Build history of the part. All positions in model axes, mm. Give positions to 0.01 mm unless a question says otherwise; leave off trailing zeros. Order: outer loops, then holes, each group sorted by start corner. A loop starts at its lowest first (then second) coordinate and runs counter-clockwise, first axis right, second up. Notation, with made-up numbers: (-22.5, -2.75) - (-1.5, -2.75) arc R27 ccw to (-1.5, 26.25) - close; hole circle Ø8 at (21.25, 11). An arc over 180 degrees is marked (long way). Use a Markdown table: item, result. Add a question column.
(1) Wall check: line 1 (X direction, y = 2.3, z = -2.5); line 2 (X direction, y = 2.25, z = -3); line 3 (Z direction, x = 6.75, y = 1.65). Give the ranges that are in metal, low to high.
(2) Slice it at D-D (x = 3). Write the cut outline in (y, z).
(3) Slice it at B-B (y = 2.6). Write the cut outline in (x, z) (3 decimals), then the cut area to 3 significant figures.
(4) Slice it at C-C (z = -13). Write the cut outline in (x, y).
(5) Mould opens along X. For faces 1 (the face through (1.44, 1.48, -2.85)), 2 (the face through (2.095, 1.479, -10.248)), 3 (the face through (7, 1, 0)) say: +X half, -X half, draft (parallel to the pull), parting line (faces both ways), or undercut.
(6) Slice it at A-A (z = -2.5). Write the cut outline in (x, y).
from build123d import *

# Parameters (mm, degrees)
SKETCH1_R           = 1.6
SKETCH1_R_2         = 4
BOSS_EXTRUDE1_DEPTH = 3
FILLET1_R           = 5


with BuildPart() as part:
    # Sketch1 → Boss-Extrude1 (new body)
    # profile 1 of 2: a face of its own
    with BuildSketch(Plane(origin=(0, 0, 0), x_dir=(1, 0, 0), z_dir=(0, 1, 0))):
        with BuildLine():
            Line((0, 5), (0, 0))
            Line((0, 0), (15, 0))
            Line((15, 0), (15, 5))
            Line((15, 5), (11.215004122, 14.482816365))
            ThreePointArc((11.215004122, 14.482816365), (11.428104918, 13.754977983), (11.5, 13))
            ThreePointArc((11.5, 13), (6.745022017, 9.071895082), (3.784995878, 14.482816365))
            Line((3.784995878, 14.482816365), (0, 5))
        make_face()
        with Locations(Location((3, 2.5, 0), (0, 0, 270))):
            Circle(SKETCH1_R, mode=Mode.SUBTRACT)
        with Locations(Location((12, 2.5, 0), (0, 0, 270))):
            Circle(SKETCH1_R, mode=Mode.SUBTRACT)
    # profile 2 of 2: a face of its own
    with BuildSketch(Plane(origin=(0, 0, 0), x_dir=(1, 0, 0), z_dir=(0, 1, 0))):
        with Locations((7.5, 13)):
            Circle(SKETCH1_R_2)
        with Locations(Location((7.5, 13, 0), (0, 0, 270))):
            Circle(SKETCH1_R, mode=Mode.SUBTRACT)
    extrude(amount=BOSS_EXTRUDE1_DEPTH)

    # Fillet1
    fillet1_edges = [part.edges().sort_by_distance(p)[0] for p in [
        (15, 1.5, -5),
        (0, 1.5, -5),
    ]]
    fillet(fillet1_edges, radius=FILLET1_R)


solid = part.part
Solution:
| question | item | result |
|---|---|---|
| 1 | line 1 | 0 to 1.4, 4.6 to 10.4, 13.6 to 15 |
| 1 | line 2 | 0 to 1.48, 4.52 to 10.48, 13.52 to 15 |
| 1 | line 3 | -16.93 to -14.41, -11.59 to 0 |
| 2 | outline | (0, -12.52) - (3, -12.52) - (3, -4.1) - (0, -4.1) - close; (0, -0.9) - (3, -0.9) - (3, 0) - (0, 0) - close |
| 3 | outline | (0, -4.039) arc R5 ccw to (0.356, -5.893) - (3.785, -14.483) arc R4 ccw to (11.215, -14.483) - (14.644, -5.893) arc R5 ccw to (15, -4.039) - (15, 0) - (0, 0) - close; hole circle Ø3.2 at (3, -2.5); hole circle Ø3.2 at (7.5, -13); hole circle Ø3.2 at (12, -2.5) |
| 3 | area | 171 mm2 |
| 4 | outline | (3.19, 0) - (5.9, 0) - (5.9, 3) - (3.19, 3) - close; (9.1, 0) - (11.81, 0) - (11.81, 3) - (9.1, 3) - close |
| 5 | face 1 | undercut |
| 5 | face 2 | -X half |
| 5 | face 3 | draft |
| 6 | outline | (0, 0) - (1.4, 0) - (1.4, 3) - (0, 3) - close; (4.6, 0) - (10.4, 0) - (10.4, 3) - (4.6, 3) - close; (13.6, 0) - (15, 0) - (15, 3) - (13.6, 3) - close |
